Geometry check sheet. Reference: the model listing, model coordinates, mm. Round coordinates to 2 decimals unless told otherwise and drop trailing zeros. Loops run counter-clockwise (first coordinate to the right, second up) from the corner with the lowest first, then second, coordinate; pieces in that order, holes last. Notation, with made-up numbers: (-5, 58.5) -> (35, 58.5) arc R16 ccw to (35, 67.5) -> close; hole circle Ø5 at (69, 46.5). An arc over 180 degrees is marked (long way). Use a Markdown table: item, result. Add a question column.
Q1. Sectioned sample at B-B, the plane x = -23.5. Enter the section's corners in (y, z).
Q2. Material ranges on L1, parallel to Z at x = -27.5, y = 3.75; L2, parallel to X at y = 1.75, z = -38; L3, parallel to Z at x = 68, y = 3.25, recorded low to high.
Q3. Sectioned sample at C-C, the plane z = -25.5. Enter the section's corners in (x, y).
Q4. Sectioned sample at A-A, the plane y = 2.75. Give the number of separate pieces and of enclosed holes in the cut face, then the cut area to 3 significant figures.
Q5. Gauge pin test, flat ends, axial feed: P1, Ø3, axis at y = 4.5, z = 52, coming from the -X side; P2, Ø3, axis at x = 71, y = 3.5, coming from the -Z side; P3, Ø2, axis at x = -26.5, y = 4, coming from the -Z side. Record the tip position at first contact, or that the pin passes through.
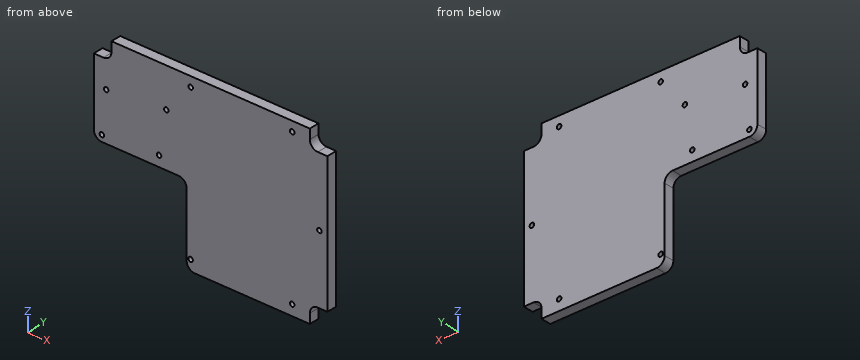
```python
from build123d import *

# Parameters (mm, degrees)
SKETCH1_R           = 1.4224
BOSS_EXTRUDE1_DEPTH = 6.35


with BuildPart() as part:
    # Sketch1 → Boss-Extrude1 (new body)
    with BuildSketch(Plane(origin=(0, 0, 0), x_dir=(1, 0, 0), z_dir=(0, 1, 0))):
        with BuildLine():
            Line((-73, -1), (-73, -43))
            Line((-73, -43), (-67, -43))
            ThreePointArc((-67, -43), (-63.464466094, -44.464466094), (-62, -48))
            Line((-62, -48), (-62, -54))
            Line((-62, -54), (62, -54))
            Line((62, -54), (62, -48))
            ThreePointArc((62, -48), (63.464466094, -44.464466094), (67, -43))
            Line((67, -43), (73, -43))
            Line((73, -43), (73, 43))
            Line((73, 43), (67, 43))
            ThreePointArc((67, 43), (63.464466094, 44.464466094), (62, 48))
            Line((62, 48), (62, 54))
            Line((62, 54), (-10, 54))
            ThreePointArc((-10, 54), (-13.535533906, 52.535533906), (-15, 49))
            Line((-15, 49), (-15, 9))
            ThreePointArc((-15, 9), (-16.464466094, 5.464466094), (-20, 4))
            Line((-20, 4), (-68, 4))
            ThreePointArc((-68, 4), (-71.535533906, 2.535533906), (-73, -1))
        make_face()
        with Locations(Location((68, 0, 0), (0, 0, 270))):
            Circle(SKETCH1_R, mode=Mode.SUBTRACT)
        with Locations(Location((-68, 0, 0), (0, 0, 270))):
            Circle(SKETCH1_R, mode=Mode.SUBTRACT)
        with Locations(Location((-27.69442531, -29.429, 0), (0, 0, 270))):
            Circle(SKETCH1_R, mode=Mode.SUBTRACT)
        with Locations(Location((-65.28642531, -26, 0), (0, 0, 270))):
            Circle(SKETCH1_R, mode=Mode.SUBTRACT)
        with Locations(Location((-32.26642531, -2.5812, 0), (0, 0, 270))):
            Circle(SKETCH1_R, mode=Mode.SUBTRACT)
        with Locations(Location((-12.52642531, -47.924899665, 0), (0, 0, 90))):
            Circle(SKETCH1_R, mode=Mode.SUBTRACT)
        with Locations(Location((50.975, -47.924899665, 0), (0, 0, 90))):
            Circle(SKETCH1_R, mode=Mode.SUBTRACT)
        with Locations(Location((-12.52642531, 47.325, 0), (0, 0, 90))):
            Circle(SKETCH1_R, mode=Mode.SUBTRACT)
        with Locations(Location((50.975, 47.325, 0), (0, 0, 90))):
            Circle(SKETCH1_R, mode=Mode.SUBTRACT)
    extrude(amount=BOSS_EXTRUDE1_DEPTH)


solid = part.part
```
Values:
| question | item | result |
|---|---|---|
| 1 | outline | (0, -4) -> (6.35, -4) -> (6.35, 54) -> (0, 54) -> close |
| 2 | L1 | -4 to 28.02, 30.84 to 54 |
| 2 | L2 | -15 to 73 |
| 2 | L3 | -43 to -1.42, 1.42 to 43 |
| 3 | outline | (-15, 0) -> (73, 0) -> (73, 6.35) -> (-15, 6.35) -> close |
| 4 | separate pieces | 1 |
| 4 | enclosed holes | 9 |
| 4 | area | 12,500 mm^2 |
| 5 | P1 | x = -62 |
| 5 | P2 | z = -43 |
| 5 | P3 | z = -4 |
